Autodesk Inventor part; units mm, degrees
ref_plane "YZ Plane" through (0, 0, 0) normal (1, 0, 0) x (0, 1, 0)
ref_plane "XZ Plane" through (0, 0, 0) normal (0, 1, 0) x (-1, 0, 0)
ref_plane "XY Plane" through (0, 0, 0) normal (0, 0, 1) x (1, 0, 0)
sketch "Sketch1" plane through (0, 0, 0) normal (0, 1, 0) x (-1, 0, 0)
  line L0 (23.5034, -42.4981) -> (-1.8966, -42.4981)
  line L1 (-1.8966, -42.4981) -> (-1.8966, 770.3019)
  line L2 (-1.8966, 770.3019) -> (23.5034, 770.3019)
  line L3 (23.5034, 770.3019) -> (23.5034, -42.4981)
  line L4 (20.3284, -39.3231) -> (1.2784, -39.3231)
  line L5 (1.2784, -39.3231) -> (1.2784, 767.1269)
  line L6 (1.2784, 767.1269) -> (20.3284, 767.1269)
  line L7 (20.3284, 767.1269) -> (20.3284, -39.3231)
  point P0 (0, 0)
  dimension "d0" = 25.4
  dimension "d1" = 812.8
  dimension "d2" = 3.175
ref_plane "Work Plane3" through (0, 0, 0) normal (0, -1, 0) x (1, 0, 0)
sketch "Sketch2" plane through (0, 0, 0) normal (0, -1, 0) x (1, 0, 0)
  line L0 (-1.2784, -39.3231) -> (-20.3284, -39.3231)
  line L1 (-20.3284, -39.3231) -> (-20.3284, 767.1269)
  line L2 (-1.2784, -39.3231) -> (-20.3284, -39.3231)
  line L3 (-20.3284, -39.3231) -> (-20.3284, 767.1269)
  line L4 (-20.3284, 767.1269) -> (-1.2784, 767.1269)
  line L5 (-1.2784, 767.1269) -> (-1.2784, -39.3231)
  point P0 (0, 0)
extrude "Extrusion3" add sketch "Sketch2" against normal blind 3.175
extrude "Extrusion5" add sketch "Sketch1" along normal blind 50.8
sketch "Sketch4" plane through (-23.5034, 0, 770.3019) normal (0, 0, 1) x (1, 0, 0)
  line L0 (0, 50.8) -> (25.4, 50.8)
  line L1 (0, 50.8) -> (3.175, 50.8)
  line L2 (3.175, 50.8) -> (25.4, 50.8)
  line L3 (25.4, 50.8) -> (22.225, 50.8)
  line L4 (22.225, 3.175) -> (22.225, 50.8)
  line L5 (3.175, 50.8) -> (22.225, 50.8)
  line L6 (22.225, 50.8) -> (22.225, 3.175)
  line L7 (22.225, 3.175) -> (3.175, 3.175)
  line L8 (3.175, 3.175) -> (3.175, 50.8)
  point P0 (23.5034, 0)
  point P1 (22.225, 0)
  dimension "d13" = 3.175
  dimension "d14" = 3.175
extrude "Extrusion6" cut sketch "Sketch4" against normal blind 1016
sketch "Sketch5" plane through (1.8966, 0, 770.3019) normal (1, 0, 0) x (0, 0, -1)
  line L0 (0, 0) -> (66.04, 0)
  line L1 (66.04, 0) -> (66.04, 25.4)
  line L2 (66.04, 25.4) -> (0, 25.4)
  line L3 (0, 25.4) -> (0, 0)
  circle A0 centre (66.04, 25.4) radius 14.2875
  point P0 (770.3019, 0)
  dimension "d17" = 66.04
  dimension "d18" = 25.4
  dimension "d19" = 28.575
extrude "Extrusion7" cut sketch "Sketch5" against normal blind 1016 contours A0 L2 L1 | L1 L2 A0
properties part number "36in Aluminum Channel"
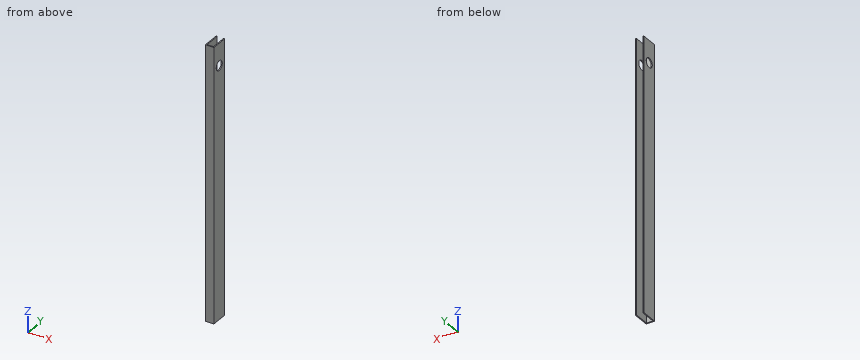
Can you work these out from the model? Positions are in its coordinate system, mm. Coordinates: 2 decimals unless noted, no trailing zeros. Write each loop counter-clockwise with the first axis right and the second up, starting at its lowest first coordinate (ties: lowest second). Pieces come first, ordered by that corner, then holes. Notation, with made-up numbers: (63, 22.25) - (90, 22.25) arc R25 cw to (90, 53.25) - close; hole circle Ø5 at (-30.75, 4.25). An arc over 180 degrees is marked (long way). Return JSON: item names as keys, results as strings.
Q1. I'm going to push flat-ended pins straight in: pin 1 Ø5.5 at (x, z) = (-10, 310) entering from +Y (3 decimals); pin 2 Ø8 at (x, y) = (-3.5, 24.5) entering from -Z. Where does each tip first touch, or does it pass through?
Computed values:
{"pin 1": "stops at y = 3.175", "pin 2": "stops at z = -42.5"}
Q2. If we section it at B-B (z = 221.5): Please give me the cut outline in (x, y) (3 decimals).
Computed values:
{"outline": "(-23.503, 0) - (1.897, 0) - (1.897, 50.8) - (-1.278, 50.8) - (-1.278, 3.175) - (-20.328, 3.175) - (-20.328, 50.8) - (-23.503, 50.8) - close"}
Q3. Please list where these lines run through material, in increasing order: L1, parallel to X at y = 28.5, z = 644.5; L2, parallel to Z at x = 0.85, y = 25.4; L3, parallel to Y at x = -4.25, z = 707.5 (3 decimals). Write a range as from..to.
Computed values:
{"L1": "x = -23.5..-20.33, -1.28..1.9", "L2": "z = -42.5..689.97, 718.55..770.3", "L3": "y = 0..3.175"}
Q4. If we section it at A-A (y = 25.4): Please give me the cut outline in (x, z).
Computed values:
{"outline": "(-23.5, -42.5) - (-20.33, -42.5) - (-20.33, 689.97) - (-23.5, 689.97) - close; (-23.5, 718.55) - (-20.33, 718.55) - (-20.33, 770.3) - (-23.5, 770.3) - close; (-1.28, -42.5) - (1.9, -42.5) - (1.9, 689.97) - (-1.28, 689.97) - close; (-1.28, 718.55) - (1.9, 718.55) - (1.9, 770.3) - (-1.28, 770.3) - close"}
